Study the drawing (mm; zero at the part's minimum x, y, z) and answer. A direction names the side the tool comes from. Give positions to 0.01 mm unless a question says otherwise; leave off trailing zeros. Loops run counter-clockwise (first coordinate to the right, second up) from the corner with the lowest first, then second, coordinate; pieces in that order, holes last. Notation, with made-up numbers: M 4.25,-9.75 L 61.25,-9.75 A20 ccw 61.25,1.25 Z; hole C -23,-37.75 d4. An arc over 180 degrees is marked long. Return JSON: item names as keys, results as strings.
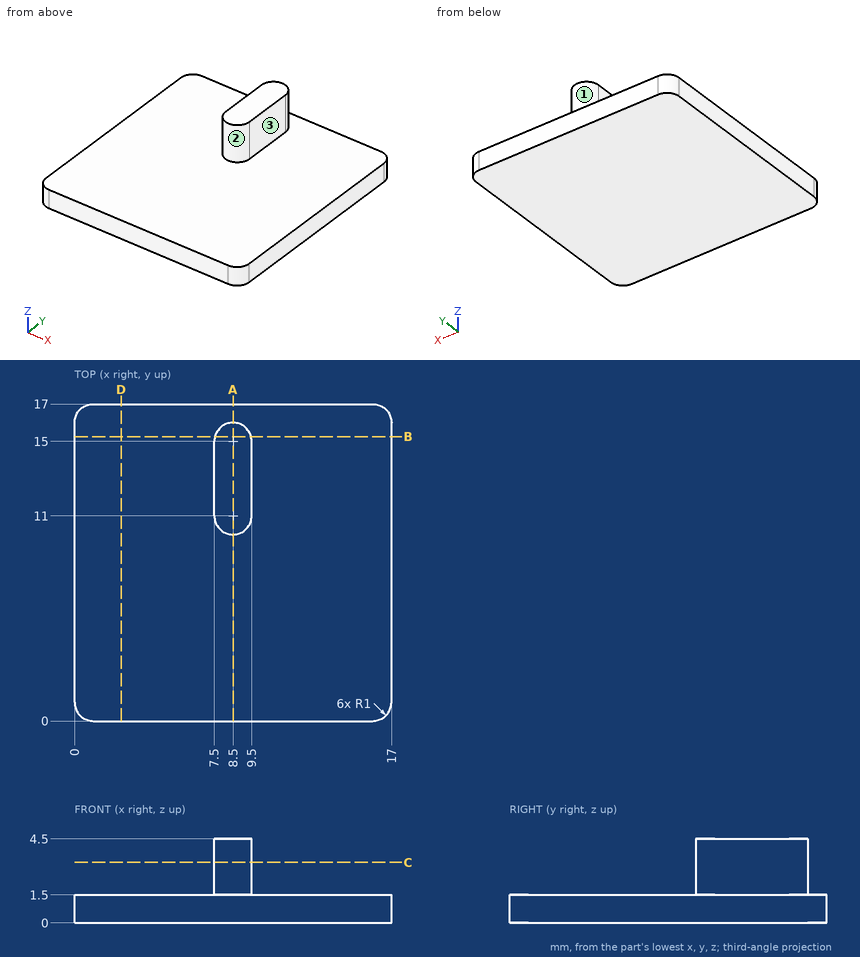
(1) The part is cut by section C-C (z = 3.25). Determine the outline of the cut face in (x, y), and give its area (3 significant figures).
Values follow:
{"outline": "M 7.5,11 A1 ccw 9.5,11 L 9.5,15 A1 ccw 7.5,15 Z", "area": "11.1 mm²"}
(2) Straight lines are drawn through the part: line 1 along X through (y, z) = (11, 3.8); line 2 along Z through (x, y) = (14, 15.25). For each, find the intervals that lie inside material, in ascending order.
Values follow:
{"line 1": "7.5 to 9.5", "line 2": "0 to 1.5"}
(3) A tool of negligible diameter and unlimited length cuts with its end or side. For the marked faces 1, 2 and 3, from which of +Z, -Z, +X, -X, +Y, -Y can it reach the whole face along a straight path? Write none if from no direction.
Values follow:
{"face 1": "+Z, +Y", "face 2": "+Z, -Y", "face 3": "+Z, +X, +Y, -Y"}
(4) The part is cut by section A-A (x = 8.5). Determine the outline of the cut face in (y, z), and give its area (3 significant figures).
Values follow:
{"outline": "M 0,0 L 17,0 L 17,1.5 L 16,1.5 L 16,4.5 L 10,4.5 L 10,1.5 L 0,1.5 Z", "area": "43.5 mm²"}
(5) Given pin 1 (1.5 mm diameter, centred on y = 12, z = 3, fed in from -X); pin 2 (2 mm diameter, centred on x = 10.5, y = 11.5, fed in from -Z); pin 3 (0.9 mm diameter, centred on y = 12.5, z = 2.5, fed in from +X); pin 4 (3 mm diameter, centred on x = 13.5, y = 15, fed in from +Z), each flat-ended and moving along its own axis, determine where each tip first touches the part or whether it passes through.
Values follow:
{"pin 1": "x = 7.5", "pin 2": "z = 0", "pin 3": "x = 9.5", "pin 4": "z = 1.5"}
(6) The part is cut by section D-D (x = 2.5). Determine the outline of the cut face in (y, z).
Values follow:
{"outline": "M 0,0 L 17,0 L 17,1.5 L 0,1.5 Z"}
(7) The part is cut by section B-B (y = 15.25). Determine the outline of the cut face in (x, z).
Values follow:
{"outline": "M 0,0 L 17,0 L 17,1.5 L 9.47,1.5 L 9.47,4.5 L 7.53,4.5 L 7.53,1.5 L 0,1.5 Z"}
